Input: part model. Units: mm. Frame: model coordinates. Give positions to 0.01 mm unless a question says otherwise; leave off trailing zeros. Order: outer loops, then holes, each group sorted by start corner. A loop starts at its lowest first (then second) coordinate and runs counter-clockwise, first axis right, second up. Notation, with made-up numbers: (69, -11) - (88, -11) arc R15 ccw to (88, 9) - close; hole circle Ø1 at (28, 69). An arc over 180 degrees is marked (long way). Use a Markdown table: item, result.
from build123d import *

# Parameters (mm, degrees)
SKETCH1_W           = 60
SKETCH1_H           = 210
BOSS_EXTRUDE1_DEPTH = 90
CUT_EXTRUDE1_REACH  = 143.51
SKETCH2_R           = 7.5


with BuildPart() as part:
    # Sketch1 → Boss-Extrude1 (new body)
    with BuildSketch(Plane.XY):
        Rectangle(SKETCH1_W, SKETCH1_H)
    extrude(amount=BOSS_EXTRUDE1_DEPTH)

    # Sketch2 → Cut-Extrude1 (cut, up to next)
    with BuildSketch(Plane.XY.offset(90), mode=Mode.PRIVATE) as cut_extrude1_sk1:
        with Locations((0, 75)):
            Circle(SKETCH2_R)
    cut_extrude1_tool1 = extrude(cut_extrude1_sk1.sketch, amount=-CUT_EXTRUDE1_REACH, mode=Mode.PRIVATE) & part.part
    # Sketch2 → Cut-Extrude1 (cut, up to next)
    with BuildSketch(Plane.XY.offset(90), mode=Mode.PRIVATE) as cut_extrude1_sk2:
        with Locations((0, -75)):
            Circle(SKETCH2_R)
    cut_extrude1_tool2 = extrude(cut_extrude1_sk2.sketch, amount=-CUT_EXTRUDE1_REACH, mode=Mode.PRIVATE) & part.part
    add(cut_extrude1_tool1.solids().sort_by_distance((0, 75, 90))[0], mode=Mode.SUBTRACT)
    add(cut_extrude1_tool2.solids().sort_by_distance((0, -75, 90))[0], mode=Mode.SUBTRACT)


solid = part.part
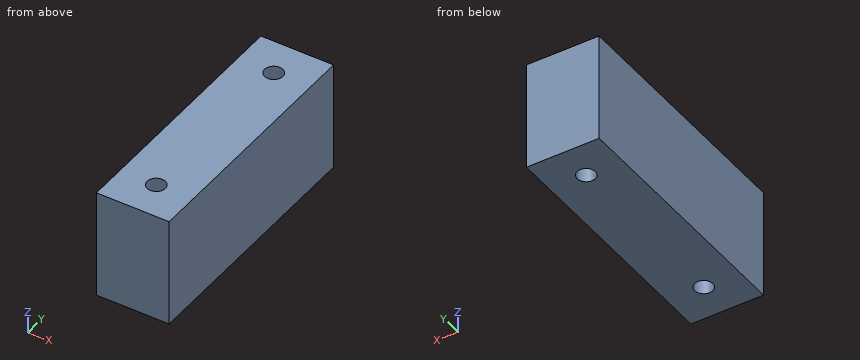
1. Section query C-C (z = 30). Return loops of the section in (x, y).
Response:
| item | result |
|---|---|
| outline | (-30, -105) - (30, -105) - (30, 105) - (-30, 105) - close; hole circle Ø15 at (0, -75); hole circle Ø15 at (0, 75) |
2. Section query A-A (x = 0). Return loops of the section in (y, z), then the cut area to 3 significant figures.
Response:
| item | result |
|---|---|
| outline | (-105, 0) - (-82.5, 0) - (-82.5, 90) - (-105, 90) - close; (-67.5, 0) - (67.5, 0) - (67.5, 90) - (-67.5, 90) - close; (82.5, 0) - (105, 0) - (105, 90) - (82.5, 90) - close |
| area | 16,200 mm^2 |
3. Material intervals for line 1 along Y through (x, z) = (0, 21.5); line 2 along Y through (x, z) = (1, 25), sorted ascending.
Response:
| item | result |
|---|---|
| line 1 | y = -105 to -82.5, -67.5 to 67.5, 82.5 to 105 |
| line 2 | y = -105 to -82.43, -67.57 to 67.57, 82.43 to 105 |
4. Section query B-B (y = -75). Return loops of the section in (x, z).
Response:
| item | result |
|---|---|
| outline | (-30, 0) - (-7.5, 0) - (-7.5, 90) - (-30, 90) - close; (7.5, 0) - (30, 0) - (30, 90) - (7.5, 90) - close |
